Print and shaded views of the part. All mm, measured from the part's lowest x, y and z. A direction names the side the tool comes from. Coordinates: 2 decimals unless noted, no trailing zeros. Write each loop counter-clockwise with the first axis right and the second up, starting at its lowest first coordinate (ties: lowest second). Pieces come first, ordered by that corner, then holes. Notation, with made-up numbers: (11, 61) -> (47, 61) arc R20 cw to (47, 76) -> close; hole circle Ø4 at (-35.5, -26). An arc over 180 degrees is marked (long way). Write item = value, one per line.
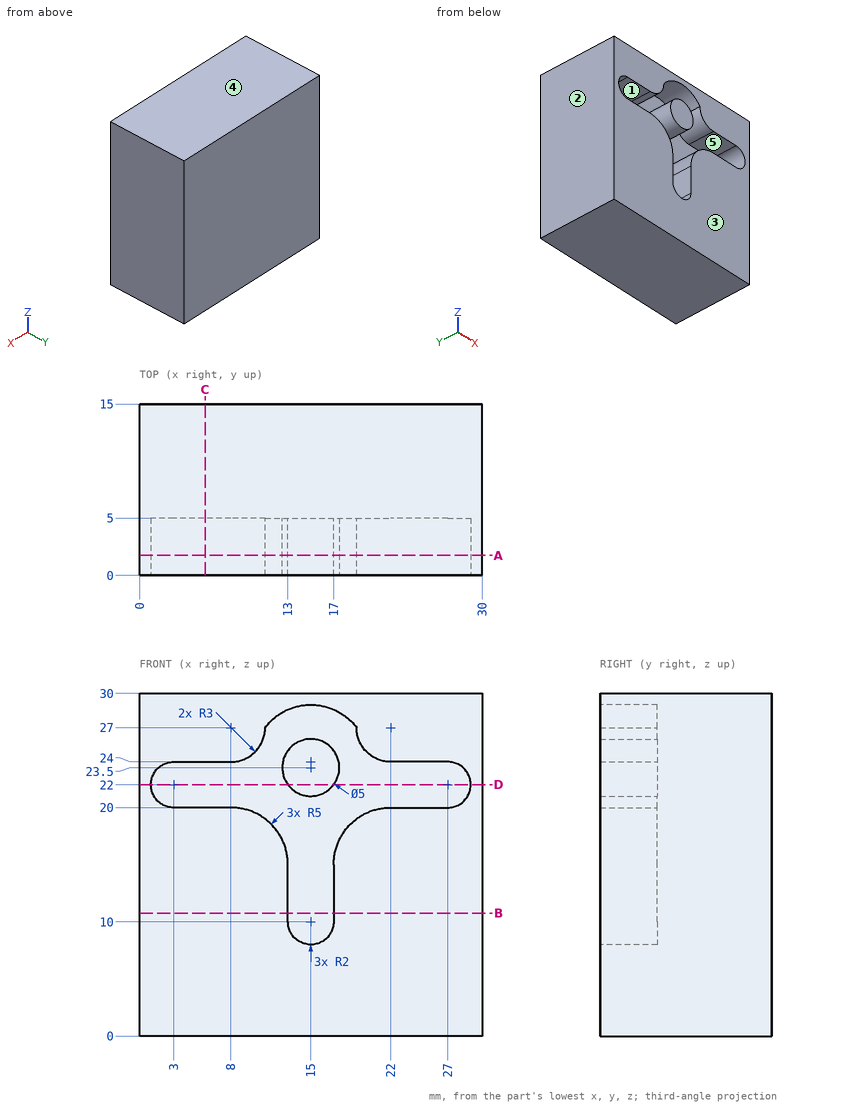
Q1. Saw through at D-D on z = 22. Give the cut face in (x, y).
Model answer:
outline = (0, 0) -> (1, 0) -> (1, 5) -> (13, 5) -> (13, 0) -> (17, 0) -> (17, 5) -> (29, 5) -> (29, 0) -> (30, 0) -> (30, 15) -> (0, 15) -> close
Q2. Probe line 1 (Z direction, x = 23.25, y = 3); line 2 (X direction, y = 3.25, z = 13); line 3 (X direction, y = 3.5, z = 27.5). List the from-to ranges inside material, lowest first. Write a range as from..to.
Model answer:
line_1 = 0..20, 24..30
line_2 = 0..13, 17..30
line_3 = 0..11.43, 18.57..30
Q3. Saw through at A-A on y = 1.75. Give the cut face in (x, z).
Model answer:
outline = (0, 0) -> (30, 0) -> (30, 30) -> (0, 30) -> close; circle Ø5 at (15, 23.5); hole (3, 20) -> (8, 20) arc R5 cw to (13, 15) -> (13, 10) arc R2 ccw to (17, 10) -> (17, 15) arc R5 cw to (22, 20) -> (27, 20) arc R2 ccw to (27, 24) -> (22, 24) arc R3 cw to (19, 27) arc R5 ccw to (11, 27) arc R3 cw to (8, 24) -> (3, 24) arc R2 ccw to start
Q4. Saw through at C-C on x = 5.75. Give the cut face in (y, z), and give its area (3 significant figures).
Model answer:
outline = (0, 0) -> (15, 0) -> (15, 30) -> (0, 30) -> (0, 24) -> (5, 24) -> (5, 20) -> (0, 20) -> close
area = 430 mm²
Q5. Saw through at B-B on z = 10.75. Give the cut face in (x, y), and give its area (3 significant figures).
Model answer:
outline = (0, 0) -> (13, 0) -> (13, 5) -> (17, 5) -> (17, 0) -> (30, 0) -> (30, 15) -> (0, 15) -> close
area = 430 mm²
Q6. Which spindle directions (+Z, -Z, +X, -X, +Y, -Y) get a long thin tool onto all of the face, cutting with end or side? Do the marked faces 1 and 2. Say none if no direction does.
Model answer:
face_1 = -Y
face_2 = +Z, -Z, -X, +Y, -Y
Q7. Mould opens along Z. For the marked faces 3, 4 and 5 say: released by +Z, released by -Z, zero draft, split by the parting line, or undercut.
Model answer:
face_3 = zero draft
face_4 = released by +Z
face_5 = undercut
